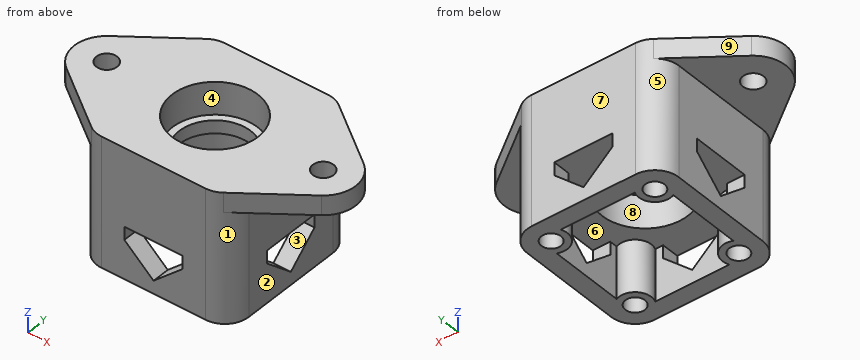
from build123d import *

# Parameters (mm, degrees)
SKETCH1_R               = 1.5
BOSS_EXTRUDE1_DEPTH     = 8
SKETCH2_R               = 5.5
BOSS_EXTRUDE2_DEPTH     = 7
SKETCH3_R               = 6.6
BOSS_EXTRUDE3_DEPTH     = 5
CUT_EXTRUDE2_DEPTH      = 33.930988446
SKETCH6_R               = 6.6
CUT_EXTRUDE3_DEPTH      = 5
BOSS_EXTRUDE4_START     = -3
SKETCH7_R               = 1.6
BOSS_EXTRUDE4_DEPTH     = 3
CIRPATTERN1_COUNT       = 2
CIRPATTERN1_ANGLE       = 90
CUT_EXTRUDE_THIN1_REACH = 33.746


with BuildPart() as part:
    # Sketch1 → Boss-Extrude1 (new body)
    with BuildSketch(Plane.XY):
        with BuildLine():
            ThreePointArc((-11.7, -8), (-10.61629509, -10.61629509), (-8, -11.7))
            Line((-8, -11.7), (8, -11.7))
            ThreePointArc((8, -11.7), (10.61629509, -10.61629509), (11.7, -8))
            Line((11.7, -8), (11.7, 8))
            ThreePointArc((11.7, 8), (10.61629509, 10.61629509), (8, 11.7))
            Line((8, 11.7), (-8, 11.7))
            ThreePointArc((-8, 11.7), (-10.61629509, 10.61629509), (-11.7, 8))
            Line((-11.7, 8), (-11.7, -8))
        make_face()
        with Locations((-8, 8)):
            Circle(SKETCH1_R, mode=Mode.SUBTRACT)
        with BuildLine():
            ThreePointArc((-8, 4.5), (-5.525126266, 5.525126266), (-4.5, 8))
            Line((-4.5, 8), (4.5, 8))
            ThreePointArc((4.5, 8), (5.525126266, 5.525126266), (8, 4.5))
            Line((8, 4.5), (8, -4.5))
            ThreePointArc((8, -4.5), (5.525126266, -5.525126266), (4.5, -8))
            Line((4.5, -8), (-4.5, -8))
            ThreePointArc((-4.5, -8), (-5.525126266, -5.525126266), (-8, -4.5))
            Line((-8, -4.5), (-8, 4.5))
        make_face(mode=Mode.SUBTRACT)
        with Locations((8, -8)):
            Circle(SKETCH1_R, mode=Mode.SUBTRACT)
        with Locations((-8, -8)):
            Circle(SKETCH1_R, mode=Mode.SUBTRACT)
        with Locations((8, 8)):
            Circle(SKETCH1_R, mode=Mode.SUBTRACT)
    extrude(amount=BOSS_EXTRUDE1_DEPTH)

    # Sketch2 → Boss-Extrude2 (add)
    with BuildSketch(Plane.XY.offset(8)):
        with BuildLine():
            Line((8, 11.7), (-8, 11.7))
            ThreePointArc((-8, 11.7), (-10.61629509, 10.61629509), (-11.7, 8))
            Line((-11.7, 8), (-11.7, -8))
            ThreePointArc((-11.7, -8), (-10.61629509, -10.61629509), (-8, -11.7))
            Line((-8, -11.7), (8, -11.7))
            ThreePointArc((8, -11.7), (10.61629509, -10.61629509), (11.7, -8))
            Line((11.7, -8), (11.7, 8))
            ThreePointArc((11.7, 8), (10.61629509, 10.61629509), (8, 11.7))
        make_face()
        Circle(SKETCH2_R, mode=Mode.SUBTRACT)
    extrude(amount=BOSS_EXTRUDE2_DEPTH)

    # Sketch3 → Boss-Extrude3 (add)
    with BuildSketch(Plane.XY.offset(15)):
        with BuildLine():
            Line((8, 11.7), (-8, 11.7))
            ThreePointArc((-8, 11.7), (-10.61629509, 10.61629509), (-11.7, 8))
            Line((-11.7, 8), (-11.7, -8))
            ThreePointArc((-11.7, -8), (-10.61629509, -10.61629509), (-8, -11.7))
            Line((-8, -11.7), (8, -11.7))
            ThreePointArc((8, -11.7), (10.61629509, -10.61629509), (11.7, -8))
            Line((11.7, -8), (11.7, 8))
            ThreePointArc((11.7, 8), (10.61629509, 10.61629509), (8, 11.7))
        make_face()
        Circle(SKETCH3_R, mode=Mode.SUBTRACT)
    extrude(amount=BOSS_EXTRUDE3_DEPTH)

    # Sketch5 → Cut-Extrude2 (cut, through all)
    with BuildSketch(Plane.XZ.offset(11.7)):
        Polygon((-4.5, 6), (0, 2), (4.5, 6), (4.5, 8), (-4.5, 8), align=None)
    cut_extrude2 = extrude(amount=-CUT_EXTRUDE2_DEPTH, mode=Mode.SUBTRACT)

    # Sketch6 → Cut-Extrude3 (cut)
    with BuildSketch(Plane(origin=(0, 0, 8), x_dir=(-1, 0, 0), z_dir=(0, 0, -1))):
        with Locations(Location((0, 0, 0), (0, 0, 180))):
            Circle(SKETCH6_R)
    extrude(amount=-CUT_EXTRUDE3_DEPTH, mode=Mode.SUBTRACT)

    # Sketch7 → Boss-Extrude4 (add)
    # profile 1 of 2: a face of its own
    with BuildSketch(Plane.XY.offset(20).offset(BOSS_EXTRUDE4_START)):
        with BuildLine():
            Line((19.659006407, 4.030419467), (10.189664741, 10.982510406))
            ThreePointArc((10.189664741, 10.982510406), (11.300890754, 9.671562212), (11.7, 8))
            Line((11.7, 8), (11.7, -8))
            ThreePointArc((11.7, -8), (11.300890754, -9.671562212), (10.189664741, -10.982510406))
            Line((10.189664741, -10.982510406), (19.659006407, -4.030419467))
            ThreePointArc((19.659006407, -4.030419467), (21.7, 0), (19.659006407, 4.030419467))
        make_face()
        with Locations((16.7, 0)):
            Circle(SKETCH7_R, mode=Mode.SUBTRACT)
    # profile 2 of 2: a face of its own
    with BuildSketch(Plane.XY.offset(20).offset(BOSS_EXTRUDE4_START)):
        with BuildLine():
            Line((-11.7, -8), (-11.7, 8))
            ThreePointArc((-11.7, 8), (-11.300890754, 9.671562212), (-10.189664741, 10.982510406))
            Line((-10.189664741, 10.982510406), (-19.659006407, 4.030419467))
            ThreePointArc((-19.659006407, 4.030419467), (-21.7, 0), (-19.659006407, -4.030419467))
            Line((-19.659006407, -4.030419467), (-10.189664741, -10.982510406))
            ThreePointArc((-10.189664741, -10.982510406), (-11.300890754, -9.671562212), (-11.7, -8))
        make_face()
        with Locations(Location((-16.7, 0, 0), (0, 0, 180))):
            Circle(SKETCH7_R, mode=Mode.SUBTRACT)
    extrude(amount=BOSS_EXTRUDE4_DEPTH)

    # CirPattern1: Cut-Extrude2 ×2 about axis
    cirpattern1_axis = Axis((0, 0, 8), (0, 0, -1))
    for i in range(1, CIRPATTERN1_COUNT):
        add(cut_extrude2.rotate(cirpattern1_axis, i * CIRPATTERN1_ANGLE / (CIRPATTERN1_COUNT - 1)), mode=Mode.SUBTRACT)

    # Cut-Extrude-Thin1: up to this face of the body (flat: up to its plane)
    cut_extrude_thin1_end = Plane(part.part.faces().sort_by_distance((-11.369074026, 0, 8))[0])
    # Sketch8 → Cut-Extrude-Thin1 (cut, up to the picked face)
    with BuildSketch(Plane(origin=(0, 0, 0), x_dir=(-1, 0, 0), z_dir=(0, 0, -1)), mode=Mode.PRIVATE) as cut_extrude_thin1_sk1:
        with BuildLine():
            Line((5.708712153, 9), (-5.708712153, 9))
            ThreePointArc((-5.708712153, 9), (-6.232233047, 6.232233047), (-9, 5.708712153))
            Line((-9, 5.708712153), (-9, -5.708712153))
            ThreePointArc((-9, -5.708712153), (-6.232233047, -6.232233047), (-5.708712153, -9))
            Line((-5.708712153, -9), (5.708712153, -9))
            ThreePointArc((5.708712153, -9), (6.232233047, -6.232233047), (9, -5.708712153))
            Line((9, -5.708712153), (9, 5.708712153))
            ThreePointArc((9, 5.708712153), (6.232233047, 6.232233047), (5.708712153, 9))
        make_face()
        with BuildLine():
            Line((4.5, 8), (-4.5, 8))
            ThreePointArc((-4.5, 8), (-5.525126266, 5.525126266), (-8, 4.5))
            Line((-8, 4.5), (-8, -4.5))
            ThreePointArc((-8, -4.5), (-5.525126266, -5.525126266), (-4.5, -8))
            Line((-4.5, -8), (4.5, -8))
            ThreePointArc((4.5, -8), (5.525126266, -5.525126266), (8, -4.5))
            Line((8, -4.5), (8, 4.5))
            ThreePointArc((8, 4.5), (5.525126266, 5.525126266), (4.5, 8))
        make_face(mode=Mode.SUBTRACT)
    cut_extrude_thin1_tool1 = split(extrude(cut_extrude_thin1_sk1.sketch, amount=-CUT_EXTRUDE_THIN1_REACH, mode=Mode.PRIVATE), bisect_by=cut_extrude_thin1_end, keep=Keep.BOTH, mode=Mode.PRIVATE)
    add(cut_extrude_thin1_tool1.solids().sort_by(Axis((-6.052233, 6.052233, 0), (0, 0, 1)))[0], mode=Mode.SUBTRACT)


solid = part.part
CAD build for the part. Positions are in the model's coordinates, mm. Face numbers are marked on the shaded views. A direction names the side the tool comes from. Round coordinates to 2 decimals unless told otherwise and drop trailing zeros. Loops run counter-clockwise (first coordinate to the right, second up) from the corner with the lowest first, then second, coordinate; pieces in that order, holes last. Notation, with made-up numbers: M 23,-34.75 L 64,-34.75 A28 ccw 64,-3.75 Z; hole C -9.75,-16 d7. An arc over 180 degrees is marked long. One line per question, with ' | ' between items. Start each with the question number.
Item 1: Cut at A-A, the plane z = 18.75. Write the cut outline in (x, y).
Item 2: Pin check, flat tips, straight feed: pin 1 Ø8 at (x, y) = (0, 0) entering from -Z; pin 2 Ø2.5 at (y, z) = (-1, 4.5) entering from -X; pin 3 Ø4 at (y, z) = (6, 15.5) entering from +X; pin 4 Ø8 at (y, z) = (2, 6) entering from +X. Stop position of each tip, or through.
Item 3: Which spindle directions (+Z, -Z, +X, -X, +Y, -Y) get a long thin tool onto all of the face, cutting with end or side? Do the marked faces 1, 2, 3, 4 and 5. Say none if no direction does.
Item 4: Wall check: line 1 (Y direction, x = 8, z = 2.5); line 2 (Y direction, x = 0, z = 14.6); line 3 (X direction, y = 4.5, z = 1.25). Give the ranges that are in metal, low to high.
Item 5: Cut at B-B, the plane x = -1. Write the cut outline in (y, z), plus the area to 3 significant figures.
Item 6: Cut at C-C, the plane y = -5. Write the cut outline in (x, z), plus the area to 3 significant figures.
Item 7: Two-plate mould, pull along X, no slides. Class the marked faces 6, 7, 8 and 9: pulls with the +X half, pulls with the -X half, needs draft (parallel to the pull), parting line crosses it, or undercut.
Item 8: Cut at D-D, the plane x = -16.7. Write the cut outline in (y, z).
Responses:
1) outline: M -19.66,-4.03 L -10.19,-10.98 A3.7 ccw -8,-11.7 L 8,-11.7 A3.7 ccw 10.19,-10.98 L 19.66,-4.03 A5 ccw 19.66,4.03 L 10.19,10.98 A3.7 ccw 8,11.7 L -8,11.7 A3.7 ccw -10.19,10.98 L -19.66,4.03 A5 ccw Z; hole C -16.7,0 d3.2; hole C 0,0 d13.2; hole C 16.7,0 d3.2
2) pin 1: passes through | pin 2: stops at x = -11.7 | pin 3: stops at x = 18.78 | pin 4: stops at x = 11.7
3) face 1: -Z, +X, -Y | face 2: -Z, +X, +Y, -Y | face 3: +X, -X | face 4: +Z | face 5: -Z, -X, +Y
4) line 1: y = -11.7 to -9.5, -6.5 to -5.5, 5.5 to 6.5, 9.5 to 11.7 | line 2: y = -11.7 to -5.5, 5.5 to 11.7 | line 3: x = -11.7 to -9, 9 to 11.7
5) outline: M -11.7,0 L -9,0 L -9,2.89 L -11.7,2.89 Z; M -11.7,8 L -6.52,8 L -6.52,13 L -5.41,13 L -5.41,15 L -6.52,15 L -6.52,20 L -11.7,20 Z; M 5.41,13 L 6.52,13 L 6.52,8 L 11.7,8 L 11.7,20 L 6.52,20 L 6.52,15 L 5.41,15 Z; M 9,0 L 11.7,0 L 11.7,2.89 L 9,2.89 Z | area: 144 mm²
6) outline: M -18.34,17 L -11.7,17 L -11.7,0 L -9,0 L -9,8 L -4.31,8 L -4.31,13 L -2.29,13 L -2.29,15 L -4.31,15 L -4.31,20 L -18.34,20 Z; M 2.29,13 L 4.31,13 L 4.31,8 L 9,8 L 9,0 L 11.7,0 L 11.7,17 L 18.34,17 L 18.34,20 L 4.31,20 L 4.31,15 L 2.29,15 Z | area: 269 mm²
7) face 6: undercut | face 7: needs draft | face 8: undercut | face 9: pulls with the -X half
8) outline: M -6.2,17 L -1.6,17 L -1.6,20 L -6.2,20 Z; M 1.6,17 L 6.2,17 L 6.2,20 L 1.6,20 Z
